Design review of the part built by this model. Coordinates are the model's own, in mm. A direction names the side the tool comes from. Give positions to 0.01 mm unless a question says otherwise; leave off trailing zeros. Order: outer loops, then holes, each group sorted by start corner. A loop starts at its lowest first (then second) coordinate and runs counter-clockwise, first axis right, second up. Notation, with made-up numbers: (83.5, 38.25) -> (112.5, 38.25) arc R33 ccw to (112.5, 73.25) -> close; hole circle Ø2 at (41, 28.25). An arc over 180 degrees is marked (long way). One line per item, written item: value. Start each with the question number.
1) Consider section B-B (z = 2.65). State how many separate pieces and enclosed holes the cut face has, plus the area to 3 significant figures.
2) Tool access review of faces 4 (the face through (5, 145, 3)), 5 (the face through (258, 60, 3)), 6 (the face through (165, 253, 3)), 7 (the face through (255, 5, 3)): name each direction out of +Z, -Z, +X, -X, +Y, -Y from which nothing blocks a thin tool from reaching the whole face with its end or side.
3) Consider section A-A (x = 59). State the section outline as (y, z) points.
4) Wall thickness on line 1 along Y through (x, z) = (130, 2.8); line 2 along X through (y, z) = (184, 5.05); line 3 along Y through (x, z) = (36, 4.15): over which ranges is each line inside the solid? List them lowest first. Write a range as from..to.
5) The part is to be moulded in two halves that separate along Y. For faces 1 (the face through (209.79, 204.18, 2.96)), 2 (the face through (95, 253, 3)), 3 (the face through (220, 250, 3)), say which applies: released by +Y, released by -Y, zero draft, split by the parting line, or undercut.
6) For pin 1 (3 mm diameter, centred on x = 218, z = 2.5, fed in from +Y); pin 2 (1.8 mm diameter, centred on y = 253, z = 4, fed in from -X); pin 3 (10 mm diameter, centred on x = 218, y = 138, fed in from -Z); pin 4 (1.8 mm diameter, centred on x = 2, z = 3, fed in from +Y), all flat-tipped, find the tip position at first contact; note any pin that passes through.
from build123d import *

# Parameters (mm, degrees)
SKIZZE1_R                       = 1.6
AUFSATZ_LINEAR_AUSTRAGEN1_DEPTH = 6


with BuildPart() as part:
    # Skizze1 → Aufsatz-Linear austragen1 (new body)
    with BuildSketch(Plane.XY):
        Polygon((35, 250), (45, 250), (45, 256), (55, 256), (55, 250), (65, 250), (65, 256), (75, 256), (75, 250), (85, 250), (85, 256), (95, 256), (95, 250), (105, 250), (105, 256), (115, 256), (115, 250), (125, 250), (125, 256), (135, 256), (135, 250), (145, 250), (145, 256), (155, 256), (155, 250), (165, 250), (165, 256), (175, 256), (175, 250), (185, 250), (185, 256), (195, 256), (195, 250), (205, 250), (205, 256), (215, 256), (215, 250), (225, 250), (255, 220), (261, 220), (261, 210), (255, 210), (255, 200), (261, 200), (261, 190), (255, 190), (255, 180), (261, 180), (261, 170), (255, 170), (255, 160), (261, 160), (261, 150), (255, 150), (255, 140), (261, 140), (261, 130), (255, 130), (255, 120), (261, 120), (261, 110), (255, 110), (255, 100), (261, 100), (261, 90), (255, 90), (255, 80), (261, 80), (261, 70), (255, 70), (255, 60), (261, 60), (261, 50), (255, 50), (255, 40), (261, 40), (261, 30), (255, 30), (255, 20), (261, 20), (261, 10), (255, 10), (255, 0), (5, 0), (5, 10), (-1, 10), (-1, 20), (5, 20), (5, 30), (-1, 30), (-1, 40), (5, 40), (5, 50), (-1, 50), (-1, 60), (5, 60), (5, 70), (-1, 70), (-1, 80), (5, 80), (5, 90), (-1, 90), (-1, 100), (5, 100), (5, 110), (-1, 110), (-1, 120), (5, 120), (5, 130), (-1, 130), (-1, 140), (5, 140), (5, 150), (-1, 150), (-1, 160), (5, 160), (5, 170), (-1, 170), (-1, 180), (5, 180), (5, 190), (-1, 190), (-1, 200), (5, 200), (5, 210), (-1, 210), (-1, 220), (5, 220), align=None)
        with Locations((20, 215)):
            Circle(SKIZZE1_R, mode=Mode.SUBTRACT)
        with Locations((30, 215)):
            Circle(SKIZZE1_R, mode=Mode.SUBTRACT)
        with Locations((240, 215)):
            Circle(SKIZZE1_R, mode=Mode.SUBTRACT)
        with Locations((230, 215)):
            Circle(SKIZZE1_R, mode=Mode.SUBTRACT)
        with Locations((20, 36)):
            Circle(SKIZZE1_R, mode=Mode.SUBTRACT)
        with Locations((130, 36)):
            Circle(SKIZZE1_R, mode=Mode.SUBTRACT)
        with Locations((240, 36)):
            Circle(SKIZZE1_R, mode=Mode.SUBTRACT)
        Polygon((65, 218.971165398), (195, 218.971165398), (225, 188.971165398), (225, 78.971165398), (35, 78.971165398), (35, 188.971165398), align=None, mode=Mode.SUBTRACT)
    extrude(amount=AUFSATZ_LINEAR_AUSTRAGEN1_DEPTH)


solid = part.part
Checked values:
1. separate pieces: 1
1. enclosed holes: 8
1. area: 37,700 mm^2
2. face 4: +Z, -Z, -X
2. face 5: +Z, -Z, +X
2. face 6: +Z, -Z, +Y
2. face 7: +Z, -Z, +X, -Y
3. outline: (0, 0) -> (78.97, 0) -> (78.97, 6) -> (0, 6) -> close; (212.97, 0) -> (250, 0) -> (250, 6) -> (212.97, 6) -> close
4. line 1: y = 0..34.4, 37.6..78.97, 218.97..256
4. line 2: x = 5..35, 225..255
4. line 3: y = 0..78.97, 189.97..250
5. face 1: undercut
5. face 2: zero draft
5. face 3: released by +Y
6. pin 1: stops at y = 250
6. pin 2: stops at x = 45
6. pin 3: passes through
6. pin 4: stops at y = 220
